from build123d import *

# Parameters (mm, degrees)
SKETCH1_W           = 18
SKETCH1_H           = 100
BOSS_EXTRUDE3_DEPTH = 18


with BuildPart() as part:
    # Sketch1 → Boss-Extrude3 (new body)
    with BuildSketch(Plane(origin=(0, 0, 0), x_dir=(0, 0, -1), z_dir=(1, 0, 0))):
        with BuildLine():
            Line((0, 0), (420, 0))
            ThreePointArc((420, 0), (490.710678119, -29.289321881), (520, -100))
            Line((520, -100), (520, -350))
            Line((520, -350), (0, -350))
            Line((0, -350), (0, -312.5))
            Line((0, -312.5), (-18, -312.5))
            Line((-18, -312.5), (-18, -212.5))
            Line((-18, -212.5), (0, -212.5))
            Line((0, -212.5), (0, -137.5))
            Line((0, -137.5), (-18, -137.5))
            Line((-18, -137.5), (-18, -37.5))
            Line((-18, -37.5), (0, -37.5))
            Line((0, -37.5), (0, 0))
        make_face()
        with Locations((260, -87.5)):
            Rectangle(SKETCH1_W, SKETCH1_H, mode=Mode.SUBTRACT)
    extrude(amount=BOSS_EXTRUDE3_DEPTH)


solid = part.part
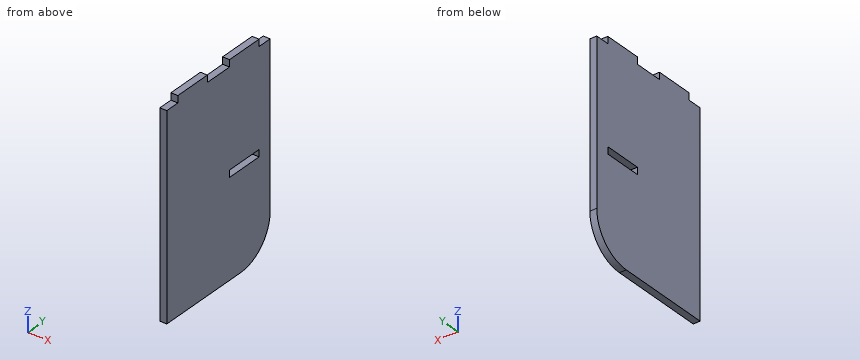
Source: CAD feature listing. Evaluate the final solid. Frame: model axes, mm. Give positions to 0.01 mm unless a question says otherwise; leave off trailing zeros. Write each loop counter-clockwise with the first axis right and the second up, starting at its lowest first coordinate (ties: lowest second). Pieces come first, ordered by that corner, then holes. Notation, with made-up numbers: M 39.5,-34.5 L 48.5,-34.5 A14 cw 48.5,-20.5 Z; hole C 54,-8.5 d2. An arc over 180 degrees is marked long. Return JSON: item names as keys, results as strings. Group by question number.
1) Cut plane D-D, the plane y = -159.5. Output: boundary loops of the cut face in (x, z), then the cut area to 3 significant figures.
2) Cut plane A-A, the plane y = -122. Output: boundary loops of the cut face in (x, z), then the cut area to 3 significant figures.
3) Ray query, L1, parallel to Z at x = 6.5, y = -108.5; L2, parallel to Z at x = 3, y = -179; L3, parallel to Y at x = 8.75, z = -260. Return the intervals inside material, ascending.
4) Cut plane B-B, the plane x = 10.5. Output: boundary loops of the cut face in (y, z).
5) First-contact query: pin 1 Ø5.5 at (x, z) = (12.5, 4.5) entering from -Y; pin 2 Ø9 at (x, y) = (11.5, -158) entering from +Z. Flat tips, straight axial feed; report the tip coordinate or a pass-through.
6) Cut plane C-C, the plane y = -65.5. Output: boundary loops of the cut face in (x, z), then the cut area to 3 significant figures.
Data:
{
 "1": {"outline": "M 0,-520 L 18,-520 L 18,0 L 0,0 Z", "area": "9,360 mm²"},
 "2": {"outline": "M 0,-520 L 18,-520 L 18,-269 L 0,-269 Z; M 0,-251 L 18,-251 L 18,18 L 0,18 Z", "area": "9,360 mm²"},
 "3": {"L1": "z = -520 to -269, -251 to 18", "L2": "z = -520 to 0", "L3": "y = -350 to -137.5, -37.5 to 0"},
 "4": {"outline": "M -350,-520 L -100,-520 A100 ccw 0,-420 L 0,0 L -37.5,0 L -37.5,18 L -137.5,18 L -137.5,0 L -212.5,0 L -212.5,18 L -312.5,18 L -312.5,0 L -350,0 Z; hole M -137.5,-269 L -37.5,-269 L -37.5,-251 L -137.5,-251 Z"},
 "5": {"pin 1": "stops at y = -312.5", "pin 2": "stops at z = 0"},
 "6": {"outline": "M 0,-513.86 L 18,-513.86 L 18,-269 L 0,-269 Z; M 0,-251 L 18,-251 L 18,18 L 0,18 Z", "area": "9,250 mm²"}
}
